Solid Edge part; units mm, degrees
sketch "Sketch1" plane through (0, 0, 0) normal (0, -1, 0) x (1, 0, 0)
  line L0 (-5.3694, 18.9) -> (-19.0694, -4.8291)
  arc A0 (-13.7, -14.1291) -> (-19.0694, -4.8291) centre (-13.7, -7.9291) cw
  line L1 (-13.7, -14.1291) -> (13.7, -14.1291)
  arc A1 (19.0694, -4.8291) -> (13.7, -14.1291) centre (13.7, -7.9291) cw
  line L2 (5.3694, 18.9) -> (19.0694, -4.8291)
  arc A2 (-5.3694, 18.9) -> (5.3694, 18.9) centre (0, 15.8) cw
  dimension "D1" = 5.3694
extrude "Protrusion1" add sketch "Sketch1" against normal blind 16
sketch "Sketch2" plane through (0, 0, 0) normal (0, -1, 0) x (1, 0, 0)
  circle A0 centre (-13.7, -7.9291) radius 2.2
  circle A1 centre (13.7, -7.9291) radius 2.2
  circle A2 centre (0, 15.8) radius 2.2
extrude "Cutout1" cut sketch "Sketch2" against normal blind 457.8755
sketch "Sketch3" plane through (0, 0, 0) normal (0, -1, 0) x (1, 0, 0)
  circle A0 centre (0, 0) radius 9.6
extrude "Cutout2" cut sketch "Sketch3" against normal blind 434.4917
sketch "Sketch4" plane through (0, 0, 3.9355) normal (0, -1, 0) x (-0.5, 0, 0.866)
  line L0 (-23.325, -5.9323) -> (-23.325, -18.9323)
  line L1 (-23.325, -18.9323) -> (16.475, -18.9323)
  line L2 (16.475, -18.9323) -> (16.475, -5.9323)
  line L3 (12.7755, -8.7037) -> (16.475, -5.9323)
  line L4 (-20.9306, -8.7037) -> (12.7755, -8.7037)
  line L5 (-20.9306, -5.9323) -> (-20.9306, -8.7037)
  line L6 (-23.325, -5.9323) -> (-20.9306, -5.9323)
  dimension "D1" = 23.325
extrude "Protrusion2" add sketch "Sketch4" against normal up to vertex (16 mm away)
sketch "Sketch5" plane through (3.1086, 0, 6.2098) normal (0, -1, 0) x (-0.5, 0, 0.866)
  line L0 (-10.3403, 2.4623) -> (-10.3403, -10.1029)
  line L1 (-10.3403, -10.1029) -> (2.6597, -10.1029)
  line L2 (2.6597, -10.1029) -> (2.6597, 2.4623)
  line L3 (2.6597, 2.4623) -> (-10.3403, 2.4623)
extrude "ExtrudedCutout_18" cut sketch "Sketch5" against normal blind 196.9446
sketch "Sketch6" plane through (13.7782, 8, 7.9355) normal (-0.866, 0, -0.5) x (0, -1, 0)
  line L0 (-2, 3.4641) -> (2, 3.4641)
  line L1 (-4, 0) -> (-2, 3.4641)
  line L2 (-2, -3.4641) -> (-4, 0)
  line L3 (2, -3.4641) -> (-2, -3.4641)
  line L4 (5.4641, 0) -> (2, -3.4641)
  line L5 (2, 3.4641) -> (5.4641, 0)
extrude "ExtrudedCutout_19" cut sketch "Sketch6" against normal blind 4
sketch "Sketch7" plane through (18.1083, 8, 10.4355) normal (0.866, 0, 0.5) x (-0.5, 0, 0.866)
  line L0 (-19.9, 8) -> (19.9, 8)
  line L1 (19.9, -8) -> (19.9, 8)
  line L2 (-19.9, -8) -> (19.9, -8)
  line L3 (-19.9, -8) -> (-19.9, 8)
extrude "ExtrudedProtrusion_14" add sketch "Sketch7" along normal blind 4
sketch "Sketch8" plane through (21.5724, 8, 12.4355) normal (0.866, 0, 0.5) x (-0.5, 0, 0.866)
  line L0 (-1.5556, 1.5556) -> (0, 3.1113)
  line L1 (0, 3.1113) -> (1.5556, 1.5556)
  arc A0 (1.5556, 1.5556) -> (-1.5556, 1.5556) centre (0, 0) cw
extrude "ExtrudedCutout_20" cut sketch "Sketch8" against normal blind 25.1595
Geometry check sheet. Reference: the model listing, model coordinates, mm. A direction names the side the tool comes from. Give positions to 0.01 mm unless a question says otherwise; leave off trailing zeros. Write each loop counter-clockwise with the first axis right and the second up, starting at its lowest first coordinate (ties: lowest second). Pieces come first, ordered by that corner, then holes.
1) Release check for a two-part mould opening along Z. For faces 1 (the flat face through (12, 16, -2)), 2 (the flat face through (22.36, 7.89, -10.09)), 3 (the cylindrical face through (19.47, 10.2, 11.14)), 4 (the flat face through (21.43, 4.33, 12.68)) record: pulls with the +Z half, pulls with the -Z half, needs draft (parallel to the pull), parting line crosses it, or undercut.
2) Section check D-D, the plane z = 15.8. Record the boundary of the cut face in (x, y).
3) Access from +Z, -Z, +X, -X, +Y, -Y to the whole of each face (thin tool, end or side, straight path). Record for faces 5 (the flat face through (16.34, 4.244, 7.442)), 6 (the flat face through (9.866, 8.112, 28.655)), 7 (the flat face through (6.76, 7.89, 11.39)).
4) Material ranges on L1, parallel to Z at x = 13, y = 11.25; L2, parallel to Z at x = 13.7, y = 5.75; L3, parallel to Z at x = 15, y = 2.75, recorded low to high.
5) Section check B-B, the plane y = 9.25. State how many separate pieces and enclosed holes the cut face has, and give its area (3 significant figures).
6) Section check A-A, the plane z = 0. Record the boundary of the cut face in (x, y).
7) Section check C-C, the plane x = 0. Record the boundary of the cut face in (y, z).
8) Gauge pin test, flat ends, axial feed: pin 1 (4 mm diameter, centred on y = 7.5, z = 8, fed in from -X); pin 2 (4 mm diameter, centred on x = -12.5, y = 8, fed in from +Z); pin 3 (6 mm diameter, centred on x = -6, y = 14.5, fed in from +Z); pin 4 (3 mm diameter, centred on x = 13, z = 19.5, fed in from -Y). Record the tip position at first contact, or that the pin passes through.
Computed:
1. face 1: needs draft
1. face 2: pulls with the -Z half
1. face 3: undercut
1. face 4: pulls with the +Z half
2. outline: (-7.16, 0) - (-2.2, 0) - (-2.2, 16) - (-7.16, 16) - close; (2.2, 0) - (19.63, 0) - (19.63, 16) - (2.2, 16) - close
3. face 5: none
3. face 6: +Z, -X, +Y, -Y
3. face 7: +Y, -Y
4. L1: z = -14.13 to -10.01, -5.84 to -0.02, 9.28 to 27.28
4. L2: z = -14.13 to -10.13, -5.73 to 0.38, 11.6 to 26.07
4. L3: z = -13.99 to -9.7, -6.15 to 1.14, 5.82 to 8.39, 8.89 to 23.82
5. separate pieces: 1
5. enclosed holes: 3
5. area: 929 mm2
6. outline: (-16.28, 0) - (-9.6, 0) - (-9.6, 16) - (-16.28, 16) - close; (13.03, 0) - (28.75, 0) - (28.75, 16) - (13.03, 16) - close
7. outline: (0, -14.13) - (16, -14.13) - (16, -9.6) - (0, -9.6) - close; (0, 9.6) - (16, 9.6) - (16, 13.6) - (0, 13.6) - close; (0, 18) - (16, 18) - (16, 22.96) - (0, 22.96) - close
8. pin 1: stops at x = -12.82
8. pin 2: stops at z = 10.01
8. pin 3: stops at z = 21.23
8. pin 4: stops at y = 0
